Work out the finished part from the listing and answer in its coordinate system (mm). Give positions to 0.01 mm unless a question says otherwise; leave off trailing zeros. Order: outer loops, then holes, each group sorted by start corner. A loop starts at its lowest first (then second) coordinate and runs counter-clockwise, first axis right, second up.
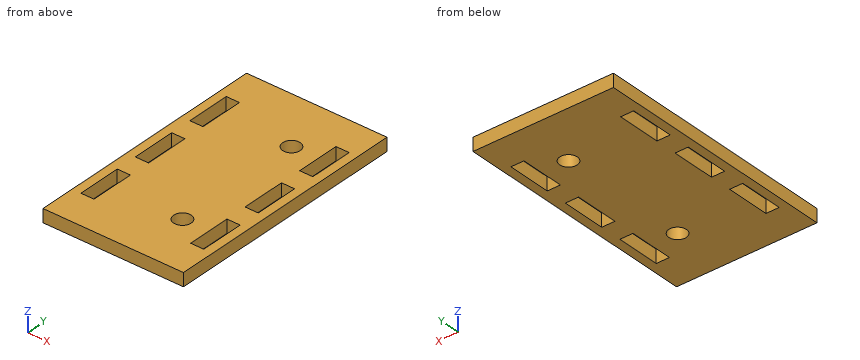
```python
from build123d import *

# Parameters (mm, degrees)
SKETCH_1_W      = 3
SKETCH_1_H      = 10
SKETCH_1_R      = 2
EXTRUDE_1_DEPTH = 3


with BuildPart() as part:
    # 草图1 → 凸台-拉伸1 (new body)
    with BuildSketch(Plane.XY):
        Polygon((25, -25), (25, 25), (25, 28), (-7, 28), (-7, 25), (-7, -25), (-7, -28), (25, -28), align=None)
        with Locations((-3.5, -15)):
            Rectangle(SKETCH_1_W, SKETCH_1_H, mode=Mode.SUBTRACT)
        with Locations((14, -15)):
            Circle(SKETCH_1_R, mode=Mode.SUBTRACT)
        with Locations((21.5, -15)):
            Rectangle(SKETCH_1_W, SKETCH_1_H, mode=Mode.SUBTRACT)
        with Locations((-3.5, 0)):
            Rectangle(SKETCH_1_W, SKETCH_1_H, mode=Mode.SUBTRACT)
        with Locations((-3.5, 15)):
            Rectangle(SKETCH_1_W, SKETCH_1_H, mode=Mode.SUBTRACT)
        with Locations((21.5, 0)):
            Rectangle(SKETCH_1_W, SKETCH_1_H, mode=Mode.SUBTRACT)
        with Locations((14, 15)):
            Circle(SKETCH_1_R, mode=Mode.SUBTRACT)
        with Locations((21.5, 15)):
            Rectangle(SKETCH_1_W, SKETCH_1_H, mode=Mode.SUBTRACT)
    extrude(amount=EXTRUDE_1_DEPTH)


solid = part.part
```
1. The part is cut by section A-A (y = -4). Write down the section's boundary in (x, z), then the cut area to 3 significant figures.
Findings below:
outline: (-7, 0) - (-5, 0) - (-5, 3) - (-7, 3) - close; (-2, 0) - (20, 0) - (20, 3) - (-2, 3) - close; (23, 0) - (25, 0) - (25, 3) - (23, 3) - close
area: 78.0 mm2
2. The part is cut by section D-D (y = -15). Write down the section's boundary in (x, z), then the cut area to 3 significant figures.
Findings below:
outline: (-7, 0) - (-5, 0) - (-5, 3) - (-7, 3) - close; (-2, 0) - (12, 0) - (12, 3) - (-2, 3) - close; (16, 0) - (20, 0) - (20, 3) - (16, 3) - close; (23, 0) - (25, 0) - (25, 3) - (23, 3) - close
area: 66.0 mm2
3. The part is cut by section B-B (z = 0.8). State how many separate pieces and enclosed holes the cut face has, then the cut area to 3 significant figures.
Findings below:
separate pieces: 1
enclosed holes: 8
area: 1,590 mm2
4. Straight lines are drawn through the part: probe 1 along X at (y, z) = (10.5, 1.65); probe 2 along Y at (x, z) = (14, 2.1); probe 3 along X at (y, z) = (-14.5, 1). For each, find the intervals that lie inside material, in ascending order.
Findings below:
probe 1: x = -7 to -5, -2 to 20, 23 to 25
probe 2: y = -28 to -17, -13 to 13, 17 to 28
probe 3: x = -7 to -5, -2 to 12.06, 15.94 to 20, 23 to 25
5. The part is cut by section C-C (x = 14). Write down the section's boundary in (y, z).
Findings below:
outline: (-28, 0) - (-17, 0) - (-17, 3) - (-28, 3) - close; (-13, 0) - (13, 0) - (13, 3) - (-13, 3) - close; (17, 0) - (28, 0) - (28, 3) - (17, 3) - close
